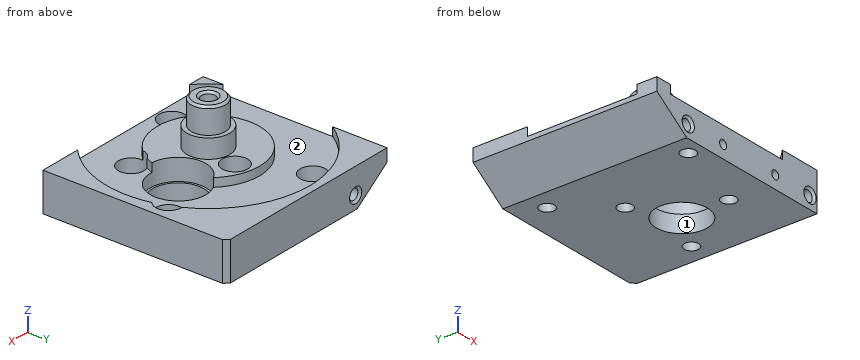
```python
from build123d import *

# Parameters (mm, degrees)
SKETCH_1_W                 = 52
SKETCH_1_H                 = 45
EXTRUDE_1_DEPTH            = 9
SKETCH_19_R                = 23.75
SKETCH_19_R_2              = 12
CUT_EXTRUDE_2_DEPTH        = 2
SKETCH_20_R                = 5
EXTRUDE_3_DEPTH            = 4.4
SKETCH_21_R                = 4
EXTRUDE_4_DEPTH            = 6
SKETCH_22_R                = 6
CUT_EXTRUDE_5_DEPTH        = 36.922277211
HOLE_WIZARD_1_D            = 3.4
HOLE_WIZARD_1_CBORE_D      = 6
HOLE_WIZARD_1_CBORE_DEPTH  = 6
CUT_EXTRUDE_6_DEPTH        = 45
HOLE_WIZARD_M3_1_D         = 2.5
HOLE_WIZARD_M3_1_DEPTH     = 9.5
HOLE_WIZARD_M3_1_TIP       = 0.751075774
HOLE_WIZARD_M4_2_D         = 3.3
HOLE_WIZARD_M4_2_DEPTH     = 10.1
HOLE_WIZARD_M4_2_TIP       = 0.991420021
CHAMFER_3_SIZE             = 0.5
M3_TAPPED_HOLE2_D          = 2.5
M3_TAPPED_HOLE2_DEPTH      = 11.5
M3_TAPPED_HOLE2_TIP        = 0.751075774
CHAMFER_4_SIZE             = 0.5
CHAMFER_5_SIZE             = 0.5
CHAMFER_6_SIZE             = 1
HOLE_WIZARD_2_D            = 3.4
HOLE_WIZARD_2_CBORE_D      = 6
HOLE_WIZARD_2_CBORE_DEPTH  = 6
EXTRUDE3_DEPTH             = 2
CHAMFER3_SIZE              = 0.5
EXTRUDE4_REACH             = 55.864
SKETCH_34_R                = 1
CUT_EXTRUDE_1_DEPTH        = 4
CUT_EXTRUDE_2_2_DEPTH      = 6
CUT_EXTRUDE_2_2_DEPTH_BACK = 3
SKETCH_35_R                = 6.5


with BuildPart() as part:
    # 草图1 → 拉伸1 (new body)
    with BuildSketch(Plane.XY):
        Rectangle(SKETCH_1_W, SKETCH_1_H)
    extrude(amount=EXTRUDE_1_DEPTH)

    # 草图19 → Cut-Extrude 2 (cut)
    with BuildSketch(Plane.XY.offset(9)):
        with Locations((0, -3)):
            Circle(SKETCH_19_R)
        with Locations((0, -3)):
            Circle(SKETCH_19_R_2, mode=Mode.SUBTRACT)
    extrude(amount=-CUT_EXTRUDE_2_DEPTH, mode=Mode.SUBTRACT)

    # 草图20 → 拉伸3 (add)
    with BuildSketch(Plane.XY.offset(9)):
        with Locations((0, -3)):
            Circle(SKETCH_20_R)
    extrude(amount=EXTRUDE_3_DEPTH)

    # 草图21 → 拉伸4 (add)
    with BuildSketch(Plane.XY.offset(13.4)):
        with Locations((0, -3)):
            Circle(SKETCH_21_R)
    extrude(amount=EXTRUDE_4_DEPTH)

    # 草图22 → 拉伸5 (cut, through all)
    with BuildSketch(Plane.XY.offset(9)):
        with Locations((11.736694594, -0.5)):
            Circle(SKETCH_22_R)
    extrude(amount=-CUT_EXTRUDE_5_DEPTH, mode=Mode.SUBTRACT)

    # 打孔尺寸根据内六角圆柱头螺钉的类型1 (through all)
    with Locations(Plane(origin=(2.210415153, 5, 9), x_dir=(1, 0, 0), z_dir=(0, 0, 1))):
        with Locations((0, 0), (9.526279441, -16.5), (19.052558883, 0)):
            CounterBoreHole(HOLE_WIZARD_1_D / 2, HOLE_WIZARD_1_CBORE_D / 2, HOLE_WIZARD_1_CBORE_DEPTH)

    # 草图25 → 拉伸6 (cut)
    with BuildSketch(Plane.XZ.offset(22.5)):
        Polygon((-26, 8), (-14.574815946, 0), (-26, 0), align=None)
    extrude(amount=-CUT_EXTRUDE_6_DEPTH, mode=Mode.SUBTRACT)

    # M3 螺纹孔1
    with Locations(Plane(origin=(-11, 22.5, 3), x_dir=(0, 0, 1), z_dir=(0, 1, 0))):
        with Locations((0, 0)):
            Hole(HOLE_WIZARD_M3_1_D / 2, depth=HOLE_WIZARD_M3_1_DEPTH)
            with Locations((0, 0, -(HOLE_WIZARD_M3_1_DEPTH + HOLE_WIZARD_M3_1_TIP / 2))):  # 118° drill point
                Cone(0, HOLE_WIZARD_M3_1_D / 2, HOLE_WIZARD_M3_1_TIP, mode=Mode.SUBTRACT)

    # M4 螺纹孔2
    with Locations(Plane(origin=(0, -3, 19.4), x_dir=(1, 0, 0), z_dir=(0, 0, 1))):
        with Locations((0, 0)):
            Hole(HOLE_WIZARD_M4_2_D / 2, depth=HOLE_WIZARD_M4_2_DEPTH)
            with Locations((0, 0, -(HOLE_WIZARD_M4_2_DEPTH + HOLE_WIZARD_M4_2_TIP / 2))):  # 118° drill point
                Cone(0, HOLE_WIZARD_M4_2_D / 2, HOLE_WIZARD_M4_2_TIP, mode=Mode.SUBTRACT)

    # 倒角3
    chamfer_3_edges = [part.edges().sort_by_distance(p)[0] for p in [
        (-4, -3, 19.4),
        (1.65, -3, 19.4),
    ]]
    chamfer(chamfer_3_edges, length=CHAMFER_3_SIZE)

    # M3 Tapped Hole2
    with Locations(Plane(origin=(-11, -22.5, 3), x_dir=(0, 0, -1), z_dir=(0, -1, 0))):
        with Locations((0, 0), (0, 35)):
            Hole(M3_TAPPED_HOLE2_D / 2, depth=M3_TAPPED_HOLE2_DEPTH)
            with Locations((0, 0, -(M3_TAPPED_HOLE2_DEPTH + M3_TAPPED_HOLE2_TIP / 2))):  # 118° drill point
                Cone(0, M3_TAPPED_HOLE2_D / 2, M3_TAPPED_HOLE2_TIP, mode=Mode.SUBTRACT)

    # 倒角4
    chamfer_4_edges = [part.edges().sort_by_distance(p)[0] for p in [
        (-11, -22.5, 1.75),
        (-11, 22.5, 4.25),
    ]]
    chamfer(chamfer_4_edges, length=CHAMFER_4_SIZE)

    # 倒角5
    chamfer_5_edges = [part.edges().sort_by_distance(p)[0] for p in [
        (24, -22.5, 1.75),
    ]]
    chamfer(chamfer_5_edges, length=CHAMFER_5_SIZE)

    # 倒角6
    chamfer_6_edges = [part.edges().sort_by_distance(p)[0] for p in [
        (26, 22.5, 4.5),
    ]]
    chamfer(chamfer_6_edges, length=CHAMFER_6_SIZE)

    # 打孔尺寸根据内六角圆柱头螺钉的类型2 (through all)
    with Locations(Plane(origin=(-6.7, 16, 9), x_dir=(1, 0, 0), z_dir=(0, 0, 1))):
        with Locations((0, 0), (0, -33)):
            CounterBoreHole(HOLE_WIZARD_2_D / 2, HOLE_WIZARD_2_CBORE_D / 2, HOLE_WIZARD_2_CBORE_DEPTH)

    # Sketch6 → Extrude3 (cut)
    with BuildSketch(Plane.XZ.offset(22.5)):
        Polygon((-26, 9), (-26, 8), (-14.574815946, 0), (26, 0), (26, 9), (13.557746863, 9), (13.557746863, 7), (-13.557746863, 7), (-13.557746863, 9), align=None)
    extrude(amount=-EXTRUDE3_DEPTH, mode=Mode.SUBTRACT)

    # Chamfer3
    chamfer3_edges = [part.edges().sort_by_distance(p)[0] for p in [
        (24, -20.5, 1.75),
        (-11, -20.5, 1.75),
    ]]
    chamfer(chamfer3_edges, length=CHAMFER3_SIZE)

    # Extrude4: up to this face of the body (flat: up to its plane)
    extrude4_end = Plane(part.part.faces().sort_by_distance((2.205978038, 22.5, 4.743303676))[0])
    # Sketch7 → Extrude4 (cut, up to the picked face)
    with BuildSketch(Plane.XZ.offset(20.5), mode=Mode.PRIVATE) as extrude4_sk1:
        Polygon((-20, 9), (-20, 6), (-11.43111196, 0), (-14.574815946, 0), (-26, 8), (-26, 9), align=None)
    extrude4_tool1 = split(extrude(extrude4_sk1.sketch, amount=-EXTRUDE4_REACH, mode=Mode.PRIVATE), bisect_by=extrude4_end, keep=Keep.BOTH, mode=Mode.PRIVATE)
    add(extrude4_tool1.solids().sort_by(Axis((-19.659359, -20.5, 5.073959), (0, 1, 0)))[0], mode=Mode.SUBTRACT)

    # 草图34 → 切除-拉伸1 (cut)
    with BuildSketch(Plane.XZ.offset(20.5)):
        with Locations(Location((-1, 3, 0), (0, 0, 270))):
            Circle(SKETCH_34_R)
        with Locations(Location((14, 3, 0), (0, 0, 270))):
            Circle(SKETCH_34_R)
    extrude(amount=-CUT_EXTRUDE_1_DEPTH, mode=Mode.SUBTRACT)

    # 草图35 → Cut-Extrude 2 2 (cut, two sides: drawn at the far end of the back side and taken through both)
    with BuildSketch(Plane.XY.offset(7).offset(-CUT_EXTRUDE_2_2_DEPTH_BACK)):
        with Locations(Location((11.736694594, -0.5, 0), (0, 0, 117.738560229))):
            Circle(SKETCH_35_R)
    extrude(amount=CUT_EXTRUDE_2_2_DEPTH + CUT_EXTRUDE_2_2_DEPTH_BACK, mode=Mode.SUBTRACT)


solid = part.part
```
Build history of the part. All positions in model axes, mm. Face numbers are marked on the shaded views. A direction names the side the tool comes from. Give positions to 0.01 mm unless a question says otherwise; leave off trailing zeros. Loops run counter-clockwise (first coordinate to the right, second up) from the corner with the lowest first, then second, coordinate; pieces in that order, holes last. Notation, with made-up numbers: (12.5, -37.5) -> (43.5, -37.5) arc R13 ccw to (43.5, -15.5) -> close; hole circle Ø2 at (-20, 21). An arc over 180 degrees is marked (long way). One line per question, with ' | ' between items. Start each with the question number.
1) Cut at C-C (x = 14). Give the cut face in (y, z).
2) 3-axis set-ups, long thin cutter, end or side, ignore diameter. For the marked faces 1 and 2: which of +Z, -Z, +X, -X, +Y, -Y reach the whole face in a straight line?
3) Cut at A-A (y = 16). Give the cut face in (x, z), plus the area to 3 significant figures.
4) Probe L1, parallel to Y at x = -6.7, z = 5.5; L2, parallel to Y at x = 14.5, z = 4.75; L3, parallel to X at y = 3.5, z = 8. List the from-to ranges inside material, lowest first.
5) Pin check, flat tips, straight feed: pin 1 (9.5 mm diameter, centred on x = -6.7, y = 16, fed in from +Z); pin 2 (1.5 mm diameter, centred on x = -2.5, z = 10, fed in from -Y); pin 3 (0.6 mm diameter, centred on x = 14, z = 3.5, fed in from -Y). Stop position of each tip, or through.
6) Cut at B-B (x = -6.7). Give the cut face in (y, z).
7) Cut at D-D (z = 10). Give the cut face in (x, y), plus the area to 3 significant figures.
Return value:
1) outline: (-20.5, 0) -> (-6.06, 0) -> (-6.06, 4) -> (-6.59, 4) -> (-6.59, 7) -> (-9.53, 7) -> (-9.53, 3) -> (-13.47, 3) -> (-13.47, 7) -> (-20.5, 7) -> (-20.5, 4) -> (-16.5, 4) -> (-16.5, 2) -> (-20.5, 2) -> close; (5.06, 0) -> (22.5, 0) -> (22.5, 9) -> (16.18, 9) -> (16.18, 7) -> (5.59, 7) -> (5.59, 4) -> (5.06, 4) -> close
2) face 1: +Z, -Z | face 2: +Z
3) outline: (-20, 6) -> (-11.43, 0) -> (-8.4, 0) -> (-8.4, 3) -> (-9.7, 3) -> (-9.7, 7) -> (-14.25, 7) -> (-14.25, 9) -> (-20, 9) -> close; (-5, 0) -> (26, 0) -> (26, 9) -> (14.25, 9) -> (14.25, 7) -> (-3.7, 7) -> (-3.7, 3) -> (-5, 3) -> close; hole circle Ø2.5 at (-11, 3) | area: 292 mm^2
4) L1: -20.5 to -20, -14 to 13, 19 to 22.5 | L2: -20.5 to -12.67, -10.33 to -6.38, 5.38 to 22.5 | L3: -10.09 to -0.39, 4.81 to 6.61, 23.86 to 26
5) pin 1: z = 9 | pin 2: y = -7.68 | pin 3: y = -16.5
6) outline: (-20.5, 0) -> (-18.7, 0) -> (-18.7, 3) -> (-20, 3) -> (-20, 7) -> (-20.5, 7) -> close; (-15.3, 0) -> (14.3, 0) -> (14.3, 3) -> (13, 3) -> (13, 7) -> (6.96, 7) -> (6.96, 9) -> (-12.96, 9) -> (-12.96, 7) -> (-14, 7) -> (-14, 3) -> (-15.3, 3) -> close; (17.7, 0) -> (22.5, 0) -> (22.5, 9) -> (19.79, 9) -> (19.79, 7) -> (19, 7) -> (19, 3) -> (17.7, 3) -> close
7) outline: circle Ø10 at (0, -3); hole circle Ø3.3 at (0, -3) | area: 70.0 mm^2
